from build123d import *

# Parameters (mm, degrees)
SKETCH1_R           = 50.8
SKETCH1_R_2         = 4.1671875
BOSS_EXTRUDE1_DEPTH = 25.4
SKETCH2_R           = 28.6512
CUT_EXTRUDE1_DEPTH  = 18.288


# Read off the part's stored shape, not the designer's step: 1/4 NPT Tapped Hole1
with BuildPart() as part:
    # Sketch1 → Boss-Extrude1 (new body)
    with BuildSketch(Plane.XY):
        Circle(SKETCH1_R)
        with Locations((-29.185832393, 29.185832393)):
            Circle(SKETCH1_R_2, mode=Mode.SUBTRACT)
        with Locations((-29.185832393, -29.185832393)):
            Circle(SKETCH1_R_2, mode=Mode.SUBTRACT)
        with Locations((29.185832393, -29.185832393)):
            Circle(SKETCH1_R_2, mode=Mode.SUBTRACT)
        with Locations((29.185832393, 29.185832393)):
            Circle(SKETCH1_R_2, mode=Mode.SUBTRACT)
    extrude(amount=BOSS_EXTRUDE1_DEPTH)

    # Sketch2 → Cut-Extrude1 (cut)
    with BuildSketch(Plane.XY.offset(25.4)):
        Circle(SKETCH2_R)
    extrude(amount=-CUT_EXTRUDE1_DEPTH, mode=Mode.SUBTRACT)

    # 1/4 NPT Tapped Hole1 outline → 1/4 NPT Tapped Hole1 (revolve, cut)
    with BuildSketch(Plane.XY.offset(12.7)):
        Polygon((6.24028647, -50.800059108), (5.943685794, -40.894), (5.5626, -40.894), (5.5626, -28.105874104), (0, -28.105874104), (0, -50.800059108), align=None)
        Polygon((0, 28.105874104), (5.5626, 28.105874104), (5.5626, 40.894), (5.943685794, 40.894), (6.2402863, 50.800053431), (0, 50.800053431), align=None)
    revolve(axis=Axis((0, 0, 12.7), (0, 1, 0)), mode=Mode.SUBTRACT)


solid = part.part
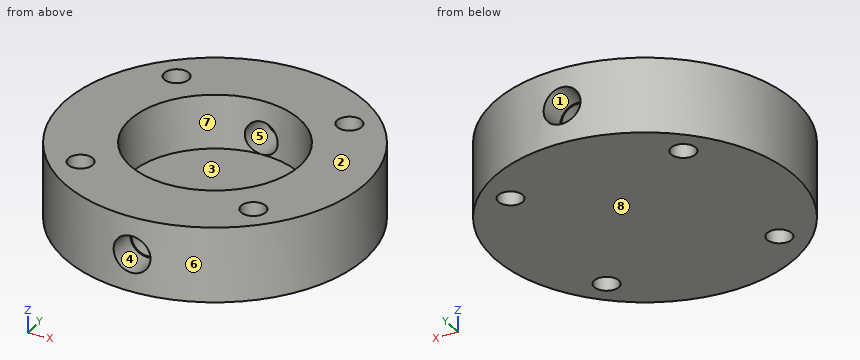
Work out the finished part from the listing and answer in its coordinate system (mm). Face numbers are marked on the shaded views. A direction names the side the tool comes from. Coordinates: 2 decimals unless noted, no trailing zeros. Write each loop counter-clockwise with the first axis right and the second up, starting at its lowest first coordinate (ties: lowest second). Pieces come first, ordered by that corner, then holes. Notation, with made-up numbers: M 73.5,-32.75 L 99.5,-32.75 A16 cw 99.5,-21.75 Z; hole C 75,30.5 d2. An arc over 180 degrees is marked long. Use one line per item in the form item = value. Start each with the question number.
1. The mould has two halves that part along X. Classify the marked faces 5, 6, 7 and 8: released by +X, released by -X, zero draft, split by the parting line, or undercut.
2. The part is cut by section D-D (z = 4.5). Give the vertices of the cut face in (x, y), plus the area to 3 significant figures.
3. Straight lines are drawn through the part: probe 1 along Y at (x, z) = (-29, 17.5); probe 2 along Z at (x, y) = (0, 37.25); probe 3 along Y at (x, z) = (-30, 6). For each, find the intervals that lie inside material, in ascending order. Write a range as from..to.
4. Each of these flat-tipped pins is pushed along its axis until it touches: P1, Ø12, axis at x = -0.5, y = 25, coming from the +Z side; P2, Ø5, axis at x = -29.19, y = 29.19, coming from the -Z side; P3, Ø4, axis at x = -16.5, z = 4, coming from the +Y side; P4, Ø3, axis at x = -13.5, z = 12.5, coming from the -Y side. Where does it stop, or does it pass through?
5. The part is cut by section B-B (x = 0). Give the number of separate pieces and of enclosed holes in the cut face, plus the area to 3 significant figures.
6. The part is cut by section C-C (y = 0). Give the vertices of the cut face in (x, z), plus the area to 3 significant figures.
7. The part is cut by section A-A (z = 12.7). Give the vertices of the cut face in (x, y), plus the area to 3 significant figures.
8. A tool of negligible diameter and unlimited length cuts with its end or side. For the marked faces 1, 2, 3 and 4, from which of +Z, -Z, +X, -X, +Y, -Y can it reach the whole face along a straight path? Write none if from no direction.
Evaluation:
q1.face_5 = undercut
q1.face_6 = split by the parting line
q1.face_7 = undercut
q1.face_8 = zero draft
q2.outline = C 0,0 d101.6; hole C -29.19,-29.19 d8.33; hole C -29.19,29.19 d8.33; hole C 29.19,-29.19 d8.33; hole C 29.19,29.19 d8.33
q2.area = 7,890 mm^2
q3.probe_1 = -41.71..-33.35, -25.02..25.02, 33.35..41.71
q3.probe_2 = 0..7.14, 18.26..25.4
q3.probe_3 = -41..-33.27, -25.1..25.1, 33.27..41
q4.P1 = 25.4
q4.P2 = through
q4.P3 = 48.69
q4.P4 = -49.36
q5.separate_pieces = 3
q5.enclosed_holes = 0
q5.area = 1,020 mm^2
q6.outline = M -50.8,0 L 50.8,0 L 50.8,25.4 L 28.65,25.4 L 28.65,7.11 L -28.65,7.11 L -28.65,25.4 L -50.8,25.4 Z
q6.area = 1,530 mm^2
q7.outline = M -6.23,-50.42 L -5.94,-40.89 L -5.56,-40.89 L -5.56,-28.11 A28.65 cw -5.56,28.11 L -5.56,40.89 L -5.94,40.89 L -6.23,50.42 A50.8 ccw Z; M 5.56,-40.89 L 5.94,-40.89 L 6.23,-50.42 A50.8 ccw 6.23,50.42 L 5.94,40.89 L 5.56,40.89 L 5.56,28.11 A28.65 cw 5.56,-28.11 Z; hole C -29.19,-29.19 d8.33; hole C -29.19,29.19 d8.33; hole C 29.19,-29.19 d8.33; hole C 29.19,29.19 d8.33
q7.area = 4,800 mm^2
q8.face_1 = +Y
q8.face_2 = +Z, +X, -X, +Y, -Y
q8.face_3 = +Z
q8.face_4 = -Y
